Verification items for the finished model (mm, model axes). A direction names the side the tool comes from. Round coordinates to 2 decimals unless told otherwise and drop trailing zeros. Order: outer loops, then holes, each group sorted by start corner. A loop starts at its lowest first (then second) coordinate and runs counter-clockwise, first axis right, second up. Notation, with made-up numbers: M 62,15 L 110,15 A30 cw 110,44 Z; hole C 47.25,43.5 d7. An arc over 180 degrees is marked long. Use CSV: the item, a comma, the result in double quotes. Start each with the question number.
Q1. Mould release check, pull along Z, two halves, no side actions. Record for faces 1 (the face through (-1, 18, -0.75)), 2 (the face through (1.4, 0, 1.4)), 3 (the face through (0, 2.5, 0)): +Z half, -Z half, draft (parallel to the pull), parting line (faces both ways), or undercut.
Q2. Gauge pin test, flat ends, axial feed: pin 1 Ø3 at (x, z) = (-2, 0.5) entering from -Y; pin 2 Ø5 at (y, z) = (4, -3) entering from +X; pin 3 Ø2 at (y, z) = (11, 0.5) entering from -X; pin 4 Ø1.5 at (x, y) = (0.5, 7) entering from -Z. Record the tip position at first contact, or that the pin passes through.
Q3. Sectioned sample at B-B (y = 13.25). Enter the section's corners in (x, z), and give its area (3 significant figures).
Q4. Scan lines: line 1 (Z direction, x = 0, y = 1.3); line 2 (Y direction, x = 2, z = 3.5); line 3 (Y direction, x = 1, z = -0.25). Record each from-to range of solid material in increasing order.
Q5. Sectioned sample at A-A (y = 5.5). Enter the section's corners in (x, z), and give its area (3 significant figures).
Q6. Set-up check for faces 4 (the face through (0, 18, -1)), 5 (the face through (0, 18, 1)), 6 (the face through (-3, 18, 0)), 7 (the face through (-2.579, 6.162, 1.978)), 8 (the face through (1.521, 17.993, -0.854)): record each of +Z, -Z, +X, -X, +Y, -Y from which the full face is reachable in a straight line by a thin tool's end or side.
```python
from build123d import *

# Parameters (mm, degrees)
SKETCH1_R           = 3.25
BOSS_EXTRUDE1_DEPTH = 12.5
SKETCH2_R           = 1.75
CUT_EXTRUDE1_DEPTH  = 2.5
SKETCH6_R           = 4.8
BOSS_EXTRUDE2_DEPTH = 5
FILLET1_R           = 0.75
BOSS_EXTRUDE3_DEPTH = 1


with BuildPart() as part:
    # Sketch1 → Boss-Extrude1 (new body)
    with BuildSketch(Plane(origin=(0, 0, 0), x_dir=(1, 0, 0), z_dir=(0, 1, 0))):
        Circle(SKETCH1_R)
    extrude(amount=BOSS_EXTRUDE1_DEPTH)

    # Sketch2 → Cut-Extrude1 (cut)
    with BuildSketch(Plane.XZ):
        Circle(SKETCH2_R)
    extrude(amount=-CUT_EXTRUDE1_DEPTH, mode=Mode.SUBTRACT)

    # Sketch6 → Boss-Extrude2 (add)
    with BuildSketch(Plane(origin=(0, 12.5, 0), x_dir=(1, 0, 0), z_dir=(0, 1, 0))):
        Circle(SKETCH6_R)
    extrude(amount=BOSS_EXTRUDE2_DEPTH)

    # Fillet1
    fillet1_edges = [part.edges().sort_by_distance(p)[0] for p in [
        (-4.8, 17.5, 0),
    ]]
    fillet(fillet1_edges, radius=FILLET1_R)

    # Sketch8 → Boss-Extrude3 (add)
    with BuildSketch(Plane(origin=(0, 17.5, 0), x_dir=(1, 0, 0), z_dir=(0, 1, 0))):
        Polygon((0, 0.75), (-3, 0.75), (-3, -0.75), (0, -0.75), (0, -1.732050808), (3, 0), (0, 1.732050808), align=None)
    extrude(amount=BOSS_EXTRUDE3_DEPTH)


solid = part.part
```
Verdict:
1,face 1,"-Z half"
1,face 2,"draft"
1,face 3,"undercut"
2,pin 1,"stops at y = 0"
2,pin 2,"stops at x = 3.21"
2,pin 3,"stops at x = -3.25"
2,pin 4,"stops at z = -3.25"
3,outline,"C 0,0 d9.6"
3,area,"72.4 mm²"
4,line 1,"z = -3.25 to -1.75, 1.75 to 3.25"
4,line 2,"y = 12.5 to 17.5"
4,line 3,"y = 2.5 to 18.5"
5,outline,"C 0,0 d6.5"
5,area,"33.2 mm²"
6,face 4,"-Z, -X, +Y"
6,face 5,"+Z, -X, +Y"
6,face 6,"+Z, -Z, -X, +Y"
6,face 7,"-Y"
6,face 8,"-Z, +X, +Y"
